```python
from build123d import *

# Parameters (mm, degrees)
SKETCH1_R           = 2
SKETCH1_R_2         = 5
BOSS_EXTRUDE1_DEPTH = 6


with BuildPart() as part:
    # Sketch1 → Boss-Extrude1 (new body)
    with BuildSketch(Plane.XY):
        with BuildLine():
            Line((-122.652649312, 114.845498823), (-69.048275573, 22))
            Line((-69.048275573, 22), (70, 22))
            Line((70, 22), (70, 47.4))
            Line((70, 47.4), (83.667882182, 56.970354135))
            ThreePointArc((83.667882182, 56.970354135), (85.235054166, 58.75737129), (85.8, 61.066114356))
            Line((85.8, 61.066114356), (85.8, 100))
            ThreePointArc((85.8, 100), (84.335533906, 103.535533906), (80.8, 105))
            Line((80.8, 105), (-18.818802154, 105))
            Line((-18.818802154, 105), (-49.04048999, 157.345498823))
            ThreePointArc((-49.04048999, 157.345498823), (-52.700744028, 161.005752861), (-57.700744028, 162.345498823))
            Line((-57.700744028, 162.345498823), (-95.228511525, 162.345498823))
            ThreePointArc((-95.228511525, 162.345498823), (-100.228511525, 161.005752861), (-103.888765563, 157.345498823))
            Line((-103.888765563, 157.345498823), (-122.652649312, 124.845498823))
            ThreePointArc((-122.652649312, 124.845498823), (-123.992395274, 119.845498823), (-122.652649312, 114.845498823))
        make_face()
        with Locations((-95.228511525, 87.345498823)):
            Circle(SKETCH1_R, mode=Mode.SUBTRACT)
        with Locations((-38.936860279, 119.845498823)):
            Circle(SKETCH1_R, mode=Mode.SUBTRACT)
        with Locations((-76.464627777, 119.845498823)):
            Circle(SKETCH1_R_2, mode=Mode.SUBTRACT)
        with Locations((-95.228511525, 152.345498823)):
            Circle(SKETCH1_R, mode=Mode.SUBTRACT)
    extrude(amount=BOSS_EXTRUDE1_DEPTH)


solid = part.part
```
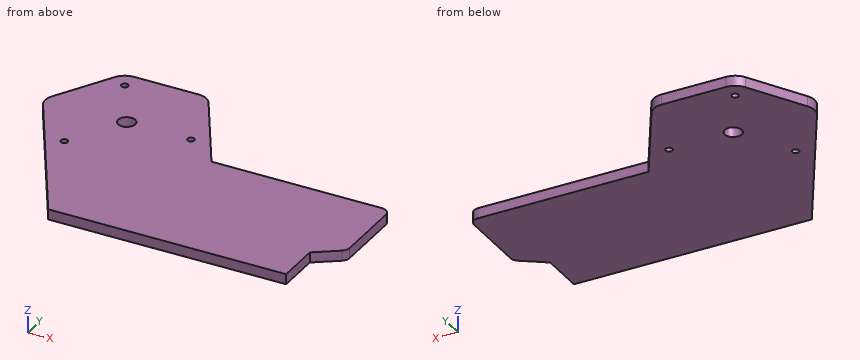
Part model, mm, in its own coordinate system. Round coordinates to 2 decimals unless told otherwise and drop trailing zeros. Loops run counter-clockwise (first coordinate to the right, second up) from the corner with the lowest first, then second, coordinate; pieces in that order, holes last. Notation, with made-up numbers: (-36, 68.25) -> (4, 68.25) arc R31 ccw to (4, 95.25) -> close; hole circle Ø8 at (26.25, 28). An arc over 180 degrees is marked (long way). Use CSV: the item, a comma, the result in double quotes. Start each with the question number.
1) Wall check: L1, parallel to X at y = 122, z = 4.8; L2, parallel to Y at x = 67, z = 0.8; L3, parallel to Y at x = -75.5, z = 0.35. Give the ranges that are in metal, low to high. Write a range as [from, to].
2) Cut at C-C, the plane y = 131. Write the cut outline in (x, z), plus the area to 3 significant figures.
3) Cut at A-A, the plane z = 5. Write the cut outline in (x, y), plus the area to 3 significant figures.
4) Cut at B-B, the plane x = 49. Write the cut outline in (y, z), plus the area to 3 significant figures.
5) Drop flat-ended pins along their axis: P1, Ø2.5, axis at x = -95.23, y = 87.35, coming from the +Z side; P2, Ø3, axis at x = -80, z = 2.5, coming from the -Y side; P3, Ø1, axis at y = 112, z = 5, coming from the -X side. Give the stop position or say it passes through.
Determined:
1,L1,"x = [-123.76, -80.98], [-71.95, -28.63]"
1,L2,"y = [22, 105]"
1,L3,"y = [33.17, 114.94], [124.75, 162.35]"
2,outline,"(-119.1, 0) -> (-33.83, 0) -> (-33.83, 6) -> (-119.1, 6) -> close"
2,area,"512 mm2"
3,outline,"(-122.65, 114.85) -> (-69.05, 22) -> (70, 22) -> (70, 47.4) -> (83.67, 56.97) arc R5 ccw to (85.8, 61.07) -> (85.8, 100) arc R5 ccw to (80.8, 105) -> (-18.82, 105) -> (-49.04, 157.35) arc R10 ccw to (-57.7, 162.35) -> (-95.23, 162.35) arc R10 ccw to (-103.89, 157.35) -> (-122.65, 124.85) arc R10 ccw to start; hole circle Ø4 at (-95.23, 87.35); hole circle Ø4 at (-95.23, 152.35); hole circle Ø10 at (-76.46, 119.85); hole circle Ø4 at (-38.94, 119.85)"
3,area,"18,800 mm2"
4,outline,"(22, 0) -> (105, 0) -> (105, 6) -> (22, 6) -> close"
4,area,"498 mm2"
5,P1,"passes through"
5,P2,"stops at y = 38.37"
5,P3,"stops at x = -121.3"
